```python
from build123d import *

# Parameters (mm, degrees)
SKETCH2_W     = 0.8
SKETCH2_H     = 0.8
CHAMFER1_SIZE = 0.2


with BuildPart() as part:
    # Sweep1: sweep along a path in Sketch1
    with BuildLine(Plane.XY) as sweep1_path:
        Line((-9.3, 0), (-1, 0))
        ThreePointArc((-1, 0), (-0.292893219, -0.292893219), (0, -1))
        Line((0, -1), (0, -7.5))
    # Sketch2 → Sweep1 (sweep)
    with BuildSketch(Plane(origin=(-9.3, 0, 0), x_dir=(0, 0, -1), z_dir=(1, 0, 0))):
        Rectangle(SKETCH2_W, SKETCH2_H)
    sweep(path=sweep1_path.line)

    # Chamfer1
    chamfer1_edges = [part.edges().sort_by_distance(p)[0] for p in [
        (0, -7.5, 0.4),
        (0.4, -7.5, 0),
        (0, -7.5, -0.4),
        (-0.4, -7.5, 0),
        (-9.3, 0.4, 0),
        (-9.3, 0, -0.4),
        (-9.3, -0.4, 0),
        (-9.3, 0, 0.4),
    ]]
    chamfer(chamfer1_edges, length=CHAMFER1_SIZE)


solid = part.part
```
The model under review builds one solid part; all positions refer to its coordinate system, in mm. Give positions to 0.01 mm unless a question says otherwise; leave off trailing zeros. Write each loop counter-clockwise with the first axis right and the second up, starting at its lowest first coordinate (ties: lowest second). Pieces come first, ordered by that corner, then holes.
(1) Consider section A-A, the plane z = 0.05. Give the boundary of the cut face in (x, y), and give its area (3 significant figures).
(2) Consider section B-B, the plane x = -6.5. Give the boundary of the cut face in (y, z), and give its area (3 significant figures).
(3) To check wall thickness, follow L1, parallel to Y at x = -1.25, z = 0.1; L2, parallel to X at y = -0.75, z = 0.25. State the ranges of each line that lie inside material, in increasing order.
Returned:
1. outline: (-9.3, -0.2) - (-9.1, -0.4) - (-1, -0.4) arc R0.6 cw to (-0.4, -1) - (-0.4, -7.3) - (-0.2, -7.5) - (0.2, -7.5) - (0.4, -7.3) - (0.4, -1) arc R1.4 ccw to (-1, 0.4) - (-9.1, 0.4) - (-9.3, 0.2) - close
1. area: 13.0 mm2
2. outline: (-0.4, -0.4) - (0.4, -0.4) - (0.4, 0.4) - (-0.4, 0.4) - close
2. area: 0.640 mm2
3. L1: y = -0.4 to 0.4
3. L2: x = -0.45 to 0.38
